from build123d import *

# Parameters (mm, degrees)
PAD_DEPTH       = 1.6
SKETCH001_R     = 2.15
POCKET_DEPTH    = 1.601
POCKET001_DEPTH = 1.601


with BuildPart() as part:
    # Sketch → Pad (new body)
    with BuildSketch(Plane.XY):
        with BuildLine():
            ThreePointArc((6.35, -6.35), (0, 0), (-6.35, -6.35))
            Line((-6.35, -6.35), (-6.35, -16.67))
            ThreePointArc((-6.35, -16.67), (0, -23.02), (6.35, -16.67))
            Line((6.35, -6.35), (6.35, -16.67))
        make_face()
    extrude(amount=PAD_DEPTH)

    # Sketch001 (on Face6 of Pad) → Pocket (cut, through all)
    with BuildSketch(Plane.XY.offset(1.6)):
        with Locations((0, -4.37)):
            Circle(SKETCH001_R)
    extrude(amount=-POCKET_DEPTH, mode=Mode.SUBTRACT)

    # Sketch002 (on Face5 of Pocket) → Pocket001 (cut, through all)
    with BuildSketch(Plane.XY.offset(1.6)):
        with BuildLine():
            ThreePointArc((2.15, -14.22), (0, -12.07), (-2.15, -14.22))
            Line((-2.15, -14.22), (-2.15, -18.59))
            ThreePointArc((-2.15, -18.59), (0, -20.74), (2.15, -18.59))
            Line((2.15, -14.22), (2.15, -18.59))
        make_face()
    extrude(amount=-POCKET001_DEPTH, mode=Mode.SUBTRACT)


solid = part.part
Here's how the part is built. I have some questions about the finished solid (model axes, mm). A direction names the side the tool comes from. Round coordinates to 2 decimals unless told otherwise and drop trailing zeros. Loops run counter-clockwise (first coordinate to the right, second up) from the corner with the lowest first, then second, coordinate; pieces in that order, holes last. Notation, with made-up numbers: M -0.5,-11 L 43.5,-11 A23 ccw 43.5,24 Z; hole C 53,75.25 d5. An arc over 180 degrees is marked long. Write each question's results on one line, items separated by ' | '. Start each with the question number.
(1) If I drill on probe 1 along Y at (x, z) = (0, 0.75); probe 2 along Y at (x, z) = (-1.5, 1.2); probe 3 along X at (y, z) = (-3, 0.2), over which ranges is the centre line in solid material (lowest first)? Write a range as from..to.
(2) Thinking about a two-plate mould opening in X: for faces 1 (the flat face through (6.35, -11, 1)), 2 (the flat face through (0, -11, 1.6)), 3 (the cylindrical face through (-0.47, -6.47, 0.81)), which applies, pulls with the +X half, pulls with the -X half, needs draft (parallel to the pull), parting line crosses it, or undercut?
(3) I want a section at D-D (y = -14). Please give me the cut outline in (x, z), then the cut area to 3 significant figures.
(4) I want a section at B-B (z = 0.4). Please give me the cut outline in (x, y), then the cut area to 3 significant figures.
(5) I want a section at A-A (x = 0). Please give me the cut outline in (y, z).
(6) I want a section at C-C (y = -4.37). Please give me the cut outline in (x, z).
(7) On a 3-axis mill with a long thin cutter (end or side, diameter ignored), from which of +Z, -Z, +X, -X, +Y, -Y can I reach the whole of each face in a straight line? I mean faces 4 (the flat face through (-6.35, -11, 1)), 5 (the cylindrical face through (-0.05, -20.74, 0.81)). Say none if no direction works.
Solved:
1) probe 1: y = -23.02..-20.74, -12.07..-6.52, -2.22..0 | probe 2: y = -22.84..-20.13, -12.68..-5.91, -2.83..-0.18 | probe 3: x = -5.39..-1.66, 1.66..5.39
2) face 1: pulls with the +X half | face 2: needs draft | face 3: undercut
3) outline: M -6.35,0 L -2.14,0 L -2.14,1.6 L -6.35,1.6 Z; M 2.14,0 L 6.35,0 L 6.35,1.6 L 2.14,1.6 Z | area: 13.5 mm²
4) outline: M -6.35,-16.67 A6.35 ccw 6.35,-16.67 L 6.35,-6.35 A6.35 ccw -6.35,-6.35 Z; hole M -2.15,-18.59 A2.15 ccw 2.15,-18.59 L 2.15,-14.22 A2.15 ccw -2.15,-14.22 Z; hole C 0,-4.37 d4.3 | area: 210 mm²
5) outline: M -23.02,0 L -20.74,0 L -20.74,1.6 L -23.02,1.6 Z; M -12.07,0 L -6.52,0 L -6.52,1.6 L -12.07,1.6 Z; M -2.22,0 L 0,0 L 0,1.6 L -2.22,1.6 Z
6) outline: M -6.03,0 L -2.15,0 L -2.15,1.6 L -6.03,1.6 Z; M 2.15,0 L 6.03,0 L 6.03,1.6 L 2.15,1.6 Z
7) face 4: +Z, -Z, -X, +Y, -Y | face 5: +Z, -Z
